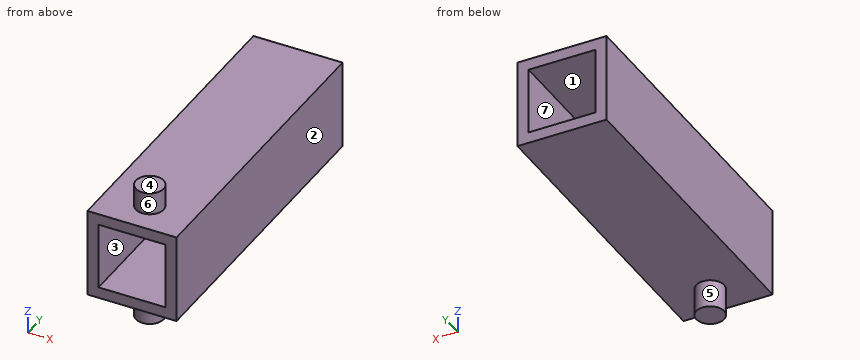
```python
from build123d import *

# Parameters (mm, degrees)
BOSS_EXTRUDE1_DEPTH      = 250
BOSS_EXTRUDE1_DEPTH_BACK = 30
SKETCH1_W                = 80
SKETCH1_H                = 80
SKETCH1_W_2              = 60
SKETCH1_H_2              = 60
SKETCH2_R                = 12.5
BOSS_EXTRUDE2_DEPTH      = 20
BOSS_EXTRUDE3_START      = 25
SKETCH3_R                = 12.5
BOSS_EXTRUDE3_DEPTH      = 25


with BuildPart() as part:
    # Sketch1 → Boss-Extrude1 (new, two sides: drawn at the far end of the back side and taken through both)
    with BuildSketch(Plane(origin=(0, 0, 0), x_dir=(1, 0, 0), z_dir=(0, 1, 0)).offset(-BOSS_EXTRUDE1_DEPTH_BACK)):
        Rectangle(SKETCH1_W, SKETCH1_H)
        Rectangle(SKETCH1_W_2, SKETCH1_H_2, mode=Mode.SUBTRACT)
    extrude(amount=BOSS_EXTRUDE1_DEPTH + BOSS_EXTRUDE1_DEPTH_BACK)

    # Sketch2 → Boss-Extrude2 (add)
    with BuildSketch(Plane.XY.offset(40)):
        Circle(SKETCH2_R)
    extrude(amount=BOSS_EXTRUDE2_DEPTH)

    # Sketch3 → Boss-Extrude3 (add)
    with BuildSketch(Plane(origin=(0, 0, -40), x_dir=(-1, 0, 0), z_dir=(0, 0, -1)).offset(BOSS_EXTRUDE3_START)):
        with Locations(Location((0, 0, 0), (0, 0, 180))):
            Circle(SKETCH3_R)
    extrude(amount=-BOSS_EXTRUDE3_DEPTH)


solid = part.part
```
The listing builds one solid part. Answer for the finished solid, in the listing's coordinates (mm). Face numbers are marked on the shaded views. A direction names the side the tool comes from. Round coordinates to 2 decimals unless told otherwise and drop trailing zeros. Write each loop counter-clockwise with the first axis right and the second up, starting at its lowest first coordinate (ties: lowest second). Pieces come first, ordered by that corner, then holes. Notation, with made-up numbers: (12.25, -20) -> (29.25, -20) arc R27 ccw to (29.25, 14) -> close; hole circle Ø8 at (-8, 60). An arc over 180 degrees is marked (long way). Answer as a JSON object with one key per item and string values. Group by question number.
Q1. Section B-B (y = 0) is taken. Write down the section's boundary in (x, z).
Q2. Straight lines are drawn through the part: line 1 along Z through (x, y) = (22, 56.5); line 2 along Z through (x, y) = (34, 235). For each, find the intervals that lie inside material, in ascending order.
Q3. Section C-C (z = 18) is taken. Write down the section's boundary in (x, y), plus the area to 3 significant figures.
Q4. Determine the mould class of the marked faces 1, 2, 3 and 4 for opening direction X: pulls with the +X half, pulls with the -X half, needs draft (parallel to the pull), parting line crosses it, or undercut.
Q5. Which of the six approach directions +Z, -Z, +X, -X, +Y, -Y give full straight-line access (tool end or side, diameter ignored) to the marked faces 5, 6 and 7?
Q6. Section D-D (x = 25) is taken. Write down the section's boundary in (y, z).
Q7. Each of these flat-tipped pins is pushed along its axis until it touches: pin 1 Ø1 at (x, y) = (1, 74.5) entering from -Z; pin 2 Ø2 at (x, z) = (-8, -47) entering from -Y; pin 3 Ø10 at (x, y) = (24.5, 109) entering from +Z. Where does it stop, or does it pass through?
Q8. Section A-A (x = 0) is taken. Write down the section's boundary in (y, z).
Check values:
{
 "1": {"outline": "(-40, -40) -> (-12.5, -40) -> (-12.5, -65) -> (12.5, -65) -> (12.5, -40) -> (40, -40) -> (40, 40) -> (12.5, 40) -> (12.5, 60) -> (-12.5, 60) -> (-12.5, 40) -> (-40, 40) -> close; hole (-30, -30) -> (30, -30) -> (30, 30) -> (-30, 30) -> close"},
 "2": {"line 1": "-40 to -30, 30 to 40", "line 2": "-40 to 40"},
 "3": {"outline": "(-40, -30) -> (-30, -30) -> (-30, 250) -> (-40, 250) -> close; (30, -30) -> (40, -30) -> (40, 250) -> (30, 250) -> close", "area": "5,600 mm^2"},
 "4": {"face 1": "undercut", "face 2": "pulls with the +X half", "face 3": "undercut", "face 4": "needs draft"},
 "5": {"face 5": "-Z", "face 6": "+Z", "face 7": "+Y, -Y"},
 "6": {"outline": "(-30, -40) -> (250, -40) -> (250, -30) -> (-30, -30) -> close; (-30, 30) -> (250, 30) -> (250, 40) -> (-30, 40) -> close"},
 "7": {"pin 1": "z = -40", "pin 2": "y = -10.36", "pin 3": "z = 40"},
 "8": {"outline": "(-30, -40) -> (-12.5, -40) -> (-12.5, -65) -> (12.5, -65) -> (12.5, -40) -> (250, -40) -> (250, -30) -> (-30, -30) -> close; (-30, 30) -> (250, 30) -> (250, 40) -> (12.5, 40) -> (12.5, 60) -> (-12.5, 60) -> (-12.5, 40) -> (-30, 40) -> close"}
}
